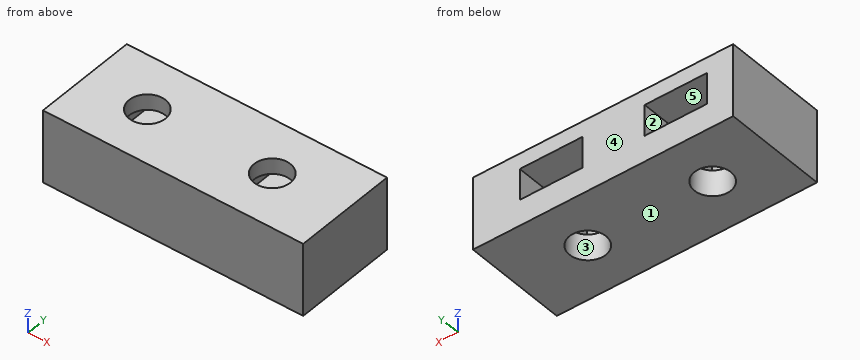
from build123d import *

# Parameters (mm, degrees)
CYLINDER028_R          = 1.75
CYLINDER028_DEPTH      = 20
CYLINDER027_R          = 1.75
CYLINDER027_DEPTH      = 20
BOX045_W               = 8
BOX045_H               = 3
BOX045_DEPTH           = 6
BOX044_W               = 8
BOX044_H               = 3
BOX044_DEPTH           = 6
BOX043_W               = 10
BOX043_H               = 7
BOX043_DEPTH           = 25
CUT044_ROLL_ANGLE      = -90
CUT044_PLACEMENT_ANGLE = 90


with BuildPart() as cylinder063:
    # Cylinder028 → Cylinder028 (new body)
    with BuildSketch(Plane(origin=(40, -18, 77), x_dir=(1, 0, 0), z_dir=(0, 0, 1))):
        Circle(CYLINDER028_R)
    extrude(amount=CYLINDER028_DEPTH)


with BuildPart() as cylinder062:
    # Cylinder027 → Cylinder027 (new body)
    with BuildSketch(Plane(origin=(28, -18, 77), x_dir=(1, 0, 0), z_dir=(0, 0, 1))):
        Circle(CYLINDER027_R)
    extrude(amount=CYLINDER027_DEPTH)


with BuildPart() as cube044:
    # Box045 → Box045 (new body)
    with BuildSketch(Plane(origin=(32, 5.5, 26.5), x_dir=(1, 0, 0), z_dir=(0, 0, 1))):
        with Locations((4, 1.5)):
            Rectangle(BOX045_W, BOX045_H)
    extrude(amount=BOX045_DEPTH)


with BuildPart() as cube043:
    # Box044 → Box044 (new body)
    with BuildSketch(Plane(origin=(32, 5.5, 38.5), x_dir=(1, 0, 0), z_dir=(0, 0, 1))):
        with Locations((4, 1.5)):
            Rectangle(BOX044_W, BOX044_H)
    extrude(amount=BOX044_DEPTH)


with BuildPart() as obj1:
    # Box043 → Box043 (new body)
    with BuildSketch(Plane(origin=(30, 4, 22), x_dir=(1, 0, 0), z_dir=(0, 0, 1))):
        with Locations((5, 3.5)):
            Rectangle(BOX043_W, BOX043_H)
    extrude(amount=BOX043_DEPTH)

    # Cut043: cut Cube043
    add(cube043.part, mode=Mode.SUBTRACT)

    # Cut044: cut Cube044
    add(cube044.part, mode=Mode.SUBTRACT)


with BuildPart() as obj1_1:
    # Cut044 roll: moved
    add(obj1.part.rotate(Axis((0, 0, 0), (1, 0, 0)), CUT044_ROLL_ANGLE))


with BuildPart() as obj1_2:
    # Cut044 placement: moved
    add(obj1_1.part.moved(Location((69, -53, 97))).rotate(Axis((69, -53, 97), (0, 0, 1)), CUT044_PLACEMENT_ANGLE))

    # Cut051: cut Cylinder062
    add(cylinder062.part, mode=Mode.SUBTRACT)

    # Cut052: cut Cylinder063
    add(cylinder063.part, mode=Mode.SUBTRACT)


with BuildPart() as obj1_3:
    # Cut052 placement: moved
    add(obj1_2.part.moved(Location((0, 0, 2))))


solid = obj1_3.part
Source: CAD feature listing. Evaluate the final solid. Frame: model axes, mm. Face numbers are marked on the shaded views. A direction names the side the tool comes from. Round coordinates to 2 decimals unless told otherwise and drop trailing zeros. Loops run counter-clockwise (first coordinate to the right, second up) from the corner with the lowest first, then second, coordinate; pieces in that order, holes last.
Q1. Access query for the marked faces 1 and 2. Directions: +Z, -Z, +X, -X, +Y, -Y. A direction counts if a zero-diameter tool reaches every point of the face in a straight line with its end or side. Return the directions, or none.
Q2. Section C-C, the plane z = 94.25. Return loops of the section in (x, y).
Q3. Section B-B, the plane y = -18. Return loops of the section in (x, z).
Q4. First-contact query: P1, Ø1.5, axis at x = 27, z = 92, coming from the +Y side. Flat tip, straight axial feed; report the tip coordinate or a pass-through.
Q5. Mould query, pull axis Y, two halves, no side actions, for the marked faces 3, 4 and 5. Classes: pulls with the +Y half, pulls with the -Y half, needs draft (parallel to the pull), parting line crosses it, or undercut.
Q6. Ray query, line 1 (X direction, y = -18, z = 94); line 2 (X direction, y = -19, z = 91.5); line 3 (Y direction, x = 40, z = 94.55). Return the intervals inside material, ascending.
Q7. Section A-A, the plane x = 28. Return loops of the section in (y, z), plus the area to 3 significant figures.
Q8. Section D-D, the plane y = -14.5. Return loops of the section in (x, z), plus the area to 3 significant figures.
Solutions:
1. face 1: -Z, +X, -X, +Y, -Y
1. face 2: +Y
2. outline: (22, -23) - (47, -23) - (47, -13) - (22, -13) - close; hole circle Ø3.5 at (28, -18); hole circle Ø3.5 at (40, -18)
3. outline: (22, 88) - (26.25, 88) - (26.25, 90.5) - (24.5, 90.5) - (24.5, 93.5) - (26.25, 93.5) - (26.25, 95) - (22, 95) - close; (29.75, 88) - (38.25, 88) - (38.25, 90.5) - (36.5, 90.5) - (36.5, 93.5) - (38.25, 93.5) - (38.25, 95) - (29.75, 95) - (29.75, 93.5) - (30.5, 93.5) - (30.5, 90.5) - (29.75, 90.5) - close; (41.75, 88) - (47, 88) - (47, 95) - (41.75, 95) - (41.75, 93.5) - (42.5, 93.5) - (42.5, 90.5) - (41.75, 90.5) - close
4. P1: stops at y = -21
5. face 3: undercut
5. face 4: pulls with the +Y half
5. face 5: needs draft
6. line 1: x = 22 to 26.25, 29.75 to 38.25, 41.75 to 47
6. line 2: x = 22 to 24.5, 30.5 to 36.5, 42.5 to 47
6. line 3: y = -23 to -19.75, -16.25 to -13
7. outline: (-23, 88) - (-19.75, 88) - (-19.75, 90.5) - (-21, 90.5) - (-21, 93.5) - (-19.75, 93.5) - (-19.75, 95) - (-23, 95) - close; (-16.25, 88) - (-13, 88) - (-13, 90.5) - (-16.25, 90.5) - close; (-16.25, 93.5) - (-13, 93.5) - (-13, 95) - (-16.25, 95) - close
7. area: 32.0 mm2
8. outline: (22, 88) - (47, 88) - (47, 95) - (22, 95) - close; hole (24.5, 90.5) - (30.5, 90.5) - (30.5, 93.5) - (24.5, 93.5) - close; hole (36.5, 90.5) - (42.5, 90.5) - (42.5, 93.5) - (36.5, 93.5) - close
8. area: 139 mm2
